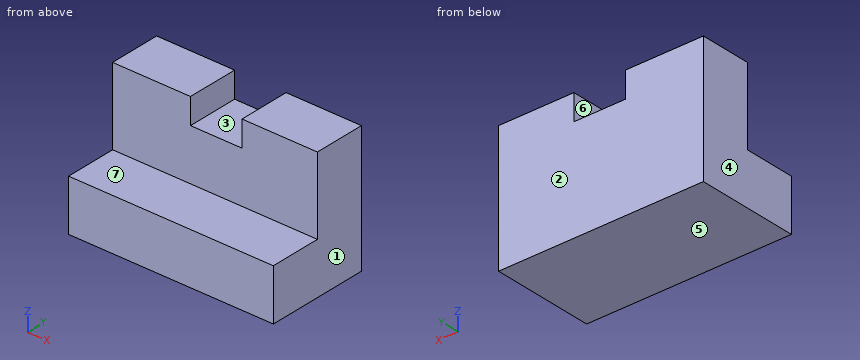
```python
from build123d import *

# Parameters (mm, degrees)
F1_DEPTH = 25.4
F2_DEPTH = 38.1
F3_W     = 12.7
F3_H     = 6.35
F4_DEPTH = 12.7
F5_W     = 13.048822
F5_H     = 19.05
F6_DEPTH = 25.4
F7_W     = 13.048822
F7_H     = 12.7
F8_DEPTH = 25.4


with BuildPart() as f1:
    # F0 (on Right) → F1 (new body)
    with BuildSketch(Plane.YZ):
        Polygon((-12.7, 0), (-12.7, -12.7), (12.7, -12.7), (12.7, 19.05), (0, 19.05), (0, 0), align=None)
    extrude(amount=F1_DEPTH)

    # F1_face (on face) → F2 (join)
    with BuildSketch(Plane(origin=(25.4, 2.721429, 0.453571), x_dir=(0, 1, 0), z_dir=(1, 0, 0))):
        Polygon((-15.421429, -0.453571), (-15.421429, -13.153571), (9.978571, -13.153571), (9.978571, 18.596429), (-2.721429, 18.596429), (-2.721429, -0.453571), align=None)
    extrude(amount=F2_DEPTH)

    # F3 (on face) → F4 (cut)
    with BuildSketch(Plane.XZ):
        with Locations((25.540019, 15.875)):
            Rectangle(F3_W, F3_H)
    extrude(amount=-F4_DEPTH, mode=Mode.SUBTRACT)

    # F5 (on face) → F6 (cut)
    with BuildSketch(Plane.XZ):
        with Locations((56.975589, 9.525)):
            Rectangle(F5_W, F5_H)
    extrude(amount=-F6_DEPTH, mode=Mode.SUBTRACT)

    # F7 (on face) → F8 (cut)
    with BuildSketch(Plane.XZ.offset(12.7)):
        with Locations((56.975589, -6.35)):
            Rectangle(F7_W, F7_H)
    extrude(amount=-F8_DEPTH, mode=Mode.SUBTRACT)


solid = f1.part
```
Here's how the part is built. I have some questions about the finished solid (model axes, mm). Face numbers are marked on the shaded views. A direction names the side the tool comes from. Round coordinates to 2 decimals unless told otherwise and drop trailing zeros. Order: outer loops, then holes, each group sorted by start corner. A loop starts at its lowest first (then second) coordinate and runs counter-clockwise, first axis right, second up. Notation, with made-up numbers: M 84,33 L 121,33 A22 ccw 121,53 Z; hole C 60.5,87 d7. An arc over 180 degrees is marked long. Answer as CSV lines item,"result".
Item 1: Please list where these lines run through material, in increasing order: L1, parallel to X at y = 10.25, z = 15; L2, parallel to Y at x = 10.5, z = 11.5; L3, parallel to Z at x = 26, y = -5. Write a range as [from, to].
From the geometry:
L1,"[0, 19.19], [31.89, 50.45]"
L2,"[0, 12.7]"
L3,"[-12.7, 0]"
Item 2: We'd pull the mould along X, two halves only. Please class the marked faces 1, 2, 3 and 4: +X half, -X half, draft (parallel to the pull), parting line (faces both ways), or undercut.
From the geometry:
face 1,"+X half"
face 2,"draft"
face 3,"undercut"
face 4,"-X half"
Item 3: Imagine slicing it at C-C on x = 14.5. List the corners of the cut face in (y, z) for me.
From the geometry:
outline,"M -12.7,-12.7 L 12.7,-12.7 L 12.7,19.05 L 0,19.05 L 0,0 L -12.7,0 Z"
Item 4: Imagine slicing it at B-B on x = 27. List the corners of the cut face in (y, z) for me.
From the geometry:
outline,"M -12.7,-12.7 L 12.7,-12.7 L 12.7,12.7 L 0,12.7 L 0,0 L -12.7,0 Z"
Item 5: Imagine slicing it at A-A on y = 7. List the corners of the cut face in (x, z) for me.
From the geometry:
outline,"M 0,-12.7 L 50.45,-12.7 L 50.45,19.05 L 31.89,19.05 L 31.89,12.7 L 19.19,12.7 L 19.19,19.05 L 0,19.05 Z"
Item 6: For pin 1 (10 mm diameter, centred on x = 25, y = 3.5, fed in from +Z); pin 2 (6 mm diameter, centred on x = 11.5, z = 14, fed in from -Y); pin 3 (6.5 mm diameter, centred on x = 35.5, y = -8, fed in from +Z), each with a flat end and sliding along its axis, tell me the tip position at first contact or that it passes through.
From the geometry:
pin 1,"z = 12.7"
pin 2,"y = 0"
pin 3,"z = 0"
Item 7: Imagine slicing it at D-D on y = -7.75. List the corners of the cut face in (x, z) for me, and give its area (3 significant figures).
From the geometry:
outline,"M 0,-12.7 L 50.45,-12.7 L 50.45,0 L 0,0 Z"
area,"641 mm2"
Item 8: Which directions (+Z, -Z, +X, -X, +Y, -Y) give clear straight access to the entire face, cutting with the end or side of a thin tool? Please do the marked faces 5, 6 and 7.
From the geometry:
face 5,"-Z, +X, -X, +Y, -Y"
face 6,"+Z, +Y, -Y"
face 7,"+Z, +X, -X, -Y"
